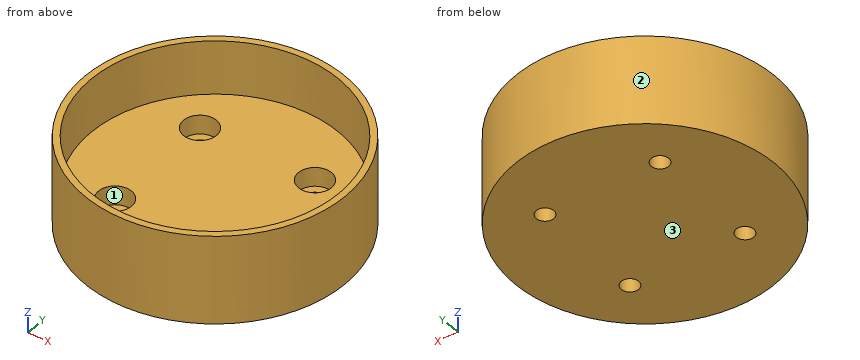
from build123d import *

# Parameters (mm, degrees)
SCHIZZO2_R                   = 41
ESTRUSIONE_ESTRUSIONE1_DEPTH = 28
SCHIZZO3_R                   = 39
TAGLIO_ESTRUSIONE1_DEPTH     = 17
SCHIZZO4_R                   = 2.75
TAGLIO_ESTRUSIONE3_DEPTH     = 29
SCHIZZO5_R                   = 5.2
TAGLIO_ESTRUSIONE4_DEPTH     = 6


with BuildPart() as part:
    # Schizzo2 → Estrusione-Estrusione1 (new body)
    with BuildSketch(Plane.XY):
        Circle(SCHIZZO2_R)
    extrude(amount=ESTRUSIONE_ESTRUSIONE1_DEPTH)

    # Schizzo3 → Taglio-Estrusione1 (cut)
    with BuildSketch(Plane.XY.offset(28)):
        Circle(SCHIZZO3_R)
    extrude(amount=-TAGLIO_ESTRUSIONE1_DEPTH, mode=Mode.SUBTRACT)

    # Schizzo4 → Taglio-Estrusione3 (cut, through all)
    with BuildSketch(Plane(origin=(0, 0, 0), x_dir=(-1, 0, 0), z_dir=(0, 0, -1))):
        with Locations((-18, 18)):
            Circle(SCHIZZO4_R)
        with Locations((18, 18)):
            Circle(SCHIZZO4_R)
        with Locations((18, -18)):
            Circle(SCHIZZO4_R)
        with Locations((-18, -18)):
            Circle(SCHIZZO4_R)
    extrude(amount=-TAGLIO_ESTRUSIONE3_DEPTH, mode=Mode.SUBTRACT)

    # Schizzo5 → Taglio-Estrusione4 (cut)
    with BuildSketch(Plane.XY.offset(11)):
        with Locations((-18, 18)):
            Circle(SCHIZZO5_R)
        with Locations((18, 18)):
            Circle(SCHIZZO5_R)
        with Locations((18, -18)):
            Circle(SCHIZZO5_R)
        with Locations((-18, -18)):
            Circle(SCHIZZO5_R)
    extrude(amount=-TAGLIO_ESTRUSIONE4_DEPTH, mode=Mode.SUBTRACT)


solid = part.part
Here's how the part is built. I have some questions about the finished solid (model axes, mm). Face numbers are marked on the shaded views. Give positions to 0.01 mm unless a question says otherwise; leave off trailing zeros. Order: outer loops, then holes, each group sorted by start corner. A loop starts at its lowest first (then second) coordinate and runs counter-clockwise, first axis right, second up. Notation, with made-up numbers: M 81,-16.75 L 94,-16.75 A29 cw 94,6.25 Z; hole C -13.5,17 d1. An arc over 180 degrees is marked long. Answer as a JSON object with one key per item and string values. Group by question number.
1) Suppose I cut it at A-A, the plane y = 18. Write out the boundary of the cut face in (x, z), plus the area to 3 significant figures.
2) I'm going to push flat-ended pins straight in: pin 1 Ø5 at (x, y) = (15.5, -17.5) entering from +Z; pin 2 Ø13.5 at (x, y) = (-18, 18) entering from +Z; pin 3 Ø6 at (y, z) = (19.5, 16.5) entering from -X. Where does each tip first touch, or does it pass through?
3) Suppose I cut it at C-C, the plane x = 0. Write out the boundary of the cut face in (y, z), plus the area to 3 significant figures.
4) We'd pull the mould along X, two halves only. Please class the marked faces 1, 2 and 3: pulls with the +X half, pulls with the -X half, needs draft (parallel to the pull), parting line crosses it, or undercut.
5) Please list where these lines run through material, in increasing order: L1, parallel to Y at x = -18, z = 3.3; L2, parallel to Y at x = 0, z = 17.5; L3, parallel to Y at x = -18, z = 6.35. Write a range as [from, to].
Results found:
{
 "1": {"outline": "M -36.84,0 L -20.75,0 L -20.75,5 L -23.2,5 L -23.2,11 L -34.6,11 L -34.6,28 L -36.84,28 Z; M -15.25,0 L 15.25,0 L 15.25,5 L 12.8,5 L 12.8,11 L -12.8,11 L -12.8,5 L -15.25,5 Z; M 20.75,0 L 36.84,0 L 36.84,28 L 34.6,28 L 34.6,11 L 23.2,11 L 23.2,5 L 20.75,5 Z", "area": "707 mm²"},
 "2": {"pin 1": "z = 5", "pin 2": "z = 11", "pin 3": "x = -37.53"},
 "3": {"outline": "M -41,0 L 41,0 L 41,28 L 39,28 L 39,11 L -39,11 L -39,28 L -41,28 Z", "area": "970 mm²"},
 "4": {"face 1": "undercut", "face 2": "parting line crosses it", "face 3": "needs draft"},
 "5": {"L1": "[-36.84, -20.75], [-15.25, 15.25], [20.75, 36.84]", "L2": "[-41, -39], [39, 41]", "L3": "[-36.84, -23.2], [-12.8, 12.8], [23.2, 36.84]"}
}
